Here's how the part is built. I have some questions about the finished solid (model axes, mm). A direction names the side the tool comes from. Give positions to 0.01 mm unless a question says otherwise; leave off trailing zeros. Loops run counter-clockwise (first coordinate to the right, second up) from the corner with the lowest first, then second, coordinate; pieces in that order, holes last. Notation, with made-up numbers: M -20.5,74 L -1.5,74 A21 cw -1.5,90 Z; hole C -15,32 d6. An arc over 180 degrees is marked long. Answer as CSV lines item,"result". Start each with the question number.
Item 1: If I drill on line 1 along Y through (x, z) = (0, 5) (3 decimals); line 2 along Y through (x, z) = (0, 16) (3 decimals); line 3 along X through (y, z) = (5, 19.5), over which ranges is the centre line in solid material (lowest first)? Write a range as from..to.
Item 2: Will these pins go through, and if not, where does the flat tip stop? P1, Ø6, axis at x = 3.5, z = 17.5, coming from the +Y side; P2, Ø1, axis at x = 8.5, z = 10, coming from the +Y side; P3, Ø10, axis at x = -10, z = 11.5, coming from the +Y side.
Item 3: For faces 4 (the cylindrical face through (-1.009, 7.684, 16.556)), 5 (the cylindrical face through (-2.799, 21.317, 1.232)), which set-ups out of +Z, -Z, +X, -X, +Y, -Y let a thin tool reach every point of the face, with its end or its side?
Item 4: I want a section at C-C on z = 15. List the corners of the cut face in (x, y) for me (3 decimals), plus the area to 3 significant figures.
Item 5: If we mould it in two halves opening along Y, with no side actions, what happens to faces 1 (the flat face through (7, -4, 20.5)), 2 (the flat face through (2, -3, 12.5)), 3 (the conical face through (-14.458, -11.086, 15.626))? For each: released by +Y, released by -Y, zero draft, split by the parting line, or undercut.
Item 6: I want a section at A-A on x = 0. List the corners of the cut face in (y, z) for me.
from build123d import *

# Parameters (mm, degrees)
SKETCH_R      = 21.5
SKETCH_R_2    = 3.35
PAD_DEPTH     = 20.5
CHAMFER_SIZE2 = 4.5
CHAMFER_SIZE  = 18
SKETCH001_R   = 7.75
POCKET_DEPTH  = 8


with BuildPart() as part:
    # Sketch → Pad (new body)
    with BuildSketch(Plane.XY):
        Circle(SKETCH_R)
        Circle(SKETCH_R_2, mode=Mode.SUBTRACT)
    extrude(amount=PAD_DEPTH)

    # Chamfer
    chamfer_edges = [part.edges().sort_by_distance(p)[0] for p in [
        (-21.5, 0, 20.5),
    ]]
    chamfer_side = part.faces().sort_by_distance((-21.5, 0, 10.25))[0]
    chamfer(chamfer_edges, length=CHAMFER_SIZE, length2=CHAMFER_SIZE2, reference=chamfer_side)

    # Sketch001 (on Face4 of Chamfer) → Pocket (cut)
    with BuildSketch(Plane.XY.offset(20.5)):
        Circle(SKETCH001_R)
    extrude(amount=-POCKET_DEPTH, mode=Mode.SUBTRACT)


solid = part.part
Result:
1,line 1,"-20.875..-3.35, 3.35..20.875"
1,line 2,"-18.125..-7.75, 7.75..18.125"
1,line 3,"-16.51..-5.92, 5.92..16.51"
2,P1,"y = 18.29"
2,P2,"y = 17.96"
2,P3,"y = 19.08"
3,face 4,"+Z"
3,face 5,"+Z, -Z"
4,outline,"C 0,0 d36.75; hole C 0,0 d15.5"
4,area,"872 mm^2"
5,face 1,"zero draft"
5,face 2,"undercut"
5,face 3,"split by the parting line"
6,outline,"M -21.5,0 L -3.35,0 L -3.35,12.5 L -7.75,12.5 L -7.75,20.5 L -17,20.5 L -21.5,2.5 Z; M 3.35,0 L 21.5,0 L 21.5,2.5 L 17,20.5 L 7.75,20.5 L 7.75,12.5 L 3.35,12.5 Z"
